Can you work these out from the drawing? Everything is in mm from the part's minimum corner. A direction names the side the tool comes from. Give positions to 0.01 mm unless a question says otherwise; leave off trailing zeros. Order: outer loops, then holes, each group sorted by start corner. A loop starts at its lowest first (then second) coordinate and runs counter-clockwise, first axis right, second up. Notation, with made-up numbers: (-2.75, -3.75) - (44.25, -3.75) arc R18 ccw to (44.25, 17.25) - close; hole circle Ø5 at (31, 82.25). An arc over 180 degrees is marked (long way). Answer as a JSON object with one key per item and string values.
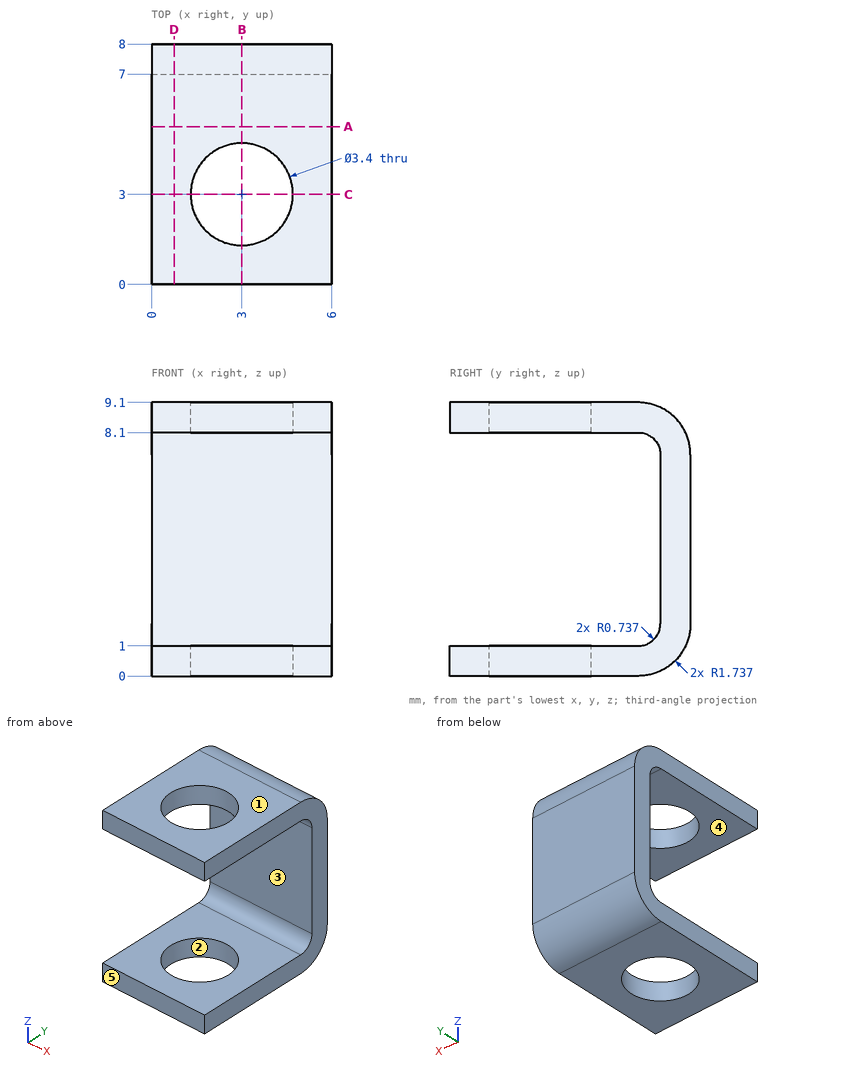
Q1. If we section it at D-D, the plane x = 0.75: Please give me the cut outline in (y, z).
Recorded:
{"outline": "(0, 0) - (6.26, 0) arc R1.74 ccw to (8, 1.74) - (8, 7.36) arc R1.74 ccw to (6.26, 9.1) - (0, 9.1) - (0, 8.1) - (6.26, 8.1) arc R0.74 cw to (7, 7.36) - (7, 1.74) arc R0.74 cw to (6.26, 1) - (0, 1) - close"}
Q2. If we section it at C-C, the plane y = 3: Please give me the cut outline in (x, z).
Recorded:
{"outline": "(0, 0) - (1.3, 0) - (1.3, 1) - (0, 1) - close; (0, 8.1) - (1.3, 8.1) - (1.3, 9.1) - (0, 9.1) - close; (4.7, 0) - (6, 0) - (6, 1) - (4.7, 1) - close; (4.7, 8.1) - (6, 8.1) - (6, 9.1) - (4.7, 9.1) - close"}
Q3. We'd pull the mould along Y, two halves only. Please class the marked faces 1, 2 and 3: released by +Y, released by -Y, zero draft, split by the parting line, or undercut.
Recorded:
{"face 1": "zero draft", "face 2": "undercut", "face 3": "released by -Y"}
Q4. Which directions (+Z, -Z, +X, -X, +Y, -Y) give clear straight access to the entire face, cutting with the end or side of a thin tool? Please do the marked faces 4 and 5.
Recorded:
{"face 4": "+X, -X, -Y", "face 5": "+Z, -Z, +X, -X, -Y"}
Q5. I need wall thicknesses on L1, parallel to Z at x = 5.75, y = 4.5; L2, parallel to Y at x = 0.8, z = 7; L3, parallel to Y at x = 3, z = 0.7 (1 decimal). Which ranges of each line are inside material? Lowest first, please.
Recorded:
{"L1": "z = 0 to 1, 8.1 to 9.1", "L2": "y = 7 to 8", "L3": "y = 0 to 1.3, 4.7 to 7.7"}
Q6. If we section it at B-B, the plane x = 3: Please give me the cut outline in (y, z).
Recorded:
{"outline": "(0, 0) - (1.3, 0) - (1.3, 1) - (0, 1) - close; (0, 8.1) - (1.3, 8.1) - (1.3, 9.1) - (0, 9.1) - close; (4.7, 0) - (6.26, 0) arc R1.74 ccw to (8, 1.74) - (8, 7.36) arc R1.74 ccw to (6.26, 9.1) - (4.7, 9.1) - (4.7, 8.1) - (6.26, 8.1) arc R0.74 cw to (7, 7.36) - (7, 1.74) arc R0.74 cw to (6.26, 1) - (4.7, 1) - close"}
Q7. I'm going to push flat-ended pins straight in: pin 1 Ø2.5 at (x, y) = (3, 3) entering from -Z; pin 2 Ø1.7 at (x, z) = (4.5, 5) entering from -Y. Where does each tip first touch, or does it pass through?
Recorded:
{"pin 1": "passes through", "pin 2": "stops at y = 7"}
Q8. If we section it at A-A, the plane y = 5.25: Please give me the cut outline in (x, z).
Recorded:
{"outline": "(0, 0) - (6, 0) - (6, 1) - (0, 1) - close; (0, 8.1) - (6, 8.1) - (6, 9.1) - (0, 9.1) - close"}
